from build123d import *

# Parameters (mm, degrees)
SKETCH2_W               = 8
SKETCH2_H               = 20
SKETCH2_W_2             = 11.75
SKETCH2_H_2             = 12.66
BOSS_EXTRUDE1_DEPTH     = 5
SKETCH3_W               = 13.1
SKETCH3_H               = 7
BOSS_EXTRUDE2_DEPTH     = 28
SKETCH4_W               = 5.75
SKETCH4_H               = 12.66
CUT_EXTRUDE1_DEPTH      = 62.587336361
SKETCH5_R               = 2
CUT_EXTRUDE2_DEPTH      = 61.902073035
SKETCH6_R               = 2
CUT_EXTRUDE3_DEPTH      = 60.059292241
SKETCH7_W               = 7
SKETCH7_H               = 28
BOSS_EXTRUDE3_DEPTH     = 19.4
SKETCH8_W               = 27
SKETCH8_H               = 33
BOSS_EXTRUDE4_DEPTH     = 2
SKETCH9_W               = 27
SKETCH9_H               = 33
BOSS_EXTRUDE5_DEPTH     = 2
CUT_EXTRUDE4_DEPTH      = 68.4388612
CUT_EXTRUDE4_DEPTH_BACK = 68.4388612


with BuildPart() as part:
    # Sketch2 → Boss-Extrude1 (new body)
    with BuildSketch(Plane(origin=(0, 0, 0), x_dir=(1, 0, 0), z_dir=(0, 1, 0))):
        with Locations((-4, 10)):
            Rectangle(SKETCH2_W, SKETCH2_H)
        Polygon((40, 0), (0, 0), (-8, 0), (-8, -7), (3.75, -7), (16.85, -7), (28.6, -7), (48, -7), (48, 0), align=None)
        with Locations((-2.125, -13.33)):
            Rectangle(SKETCH2_W_2, SKETCH2_H_2)
        with Locations((22.725, -13.33)):
            Rectangle(SKETCH2_W_2, SKETCH2_H_2)
        with Locations((44, 10)):
            Rectangle(SKETCH2_W, SKETCH2_H)
    extrude(amount=BOSS_EXTRUDE1_DEPTH)

    # Sketch3 → Boss-Extrude2 (add)
    with BuildSketch(Plane.XZ):
        Polygon((3.75, 19.66), (-8, 19.66), (-8, 0), (0, 0), (3.75, 0), (3.75, 7), align=None)
        with Locations((10.3, 3.5)):
            Rectangle(SKETCH3_W, SKETCH3_H)
        Polygon((16.85, 19.66), (16.85, 7), (16.85, 0), (28.6, 0), (28.6, 7), (28.6, 19.66), align=None)
    extrude(amount=BOSS_EXTRUDE2_DEPTH)

    # Sketch4 → Cut-Extrude1 (cut, through all)
    with BuildSketch(Plane.XZ.offset(28)):
        with Locations((-5.125, 13.33)):
            Rectangle(SKETCH4_W, SKETCH4_H)
        with Locations((25.725, 13.33)):
            Rectangle(SKETCH4_W, SKETCH4_H)
    extrude(amount=-CUT_EXTRUDE1_DEPTH, mode=Mode.SUBTRACT)

    # Sketch5 → Cut-Extrude2 (cut, through all)
    with BuildSketch(Plane.ZY.offset(2.25)):
        with Locations((13.33, -2)):
            Circle(SKETCH5_R)
        with Locations((13.33, -21)):
            Circle(SKETCH5_R)
        with Locations((13.33, -11.5)):
            Circle(SKETCH5_R)
    extrude(amount=-CUT_EXTRUDE2_DEPTH, mode=Mode.SUBTRACT)

    # Sketch6 → Cut-Extrude3 (cut, through all)
    with BuildSketch(Plane.XZ):
        with Locations(Location((43.95, -5, 0), (0, 0, 270))):
            Circle(SKETCH6_R)
        with Locations(Location((43.95, -15, 0), (0, 0, 270))):
            Circle(SKETCH6_R)
        with Locations(Location((-3.95, -5, 0), (0, 0, 270))):
            Circle(SKETCH6_R)
        with Locations(Location((-3.95, -15, 0), (0, 0, 270))):
            Circle(SKETCH6_R)
    extrude(amount=-CUT_EXTRUDE3_DEPTH, mode=Mode.SUBTRACT)

    # Sketch7 → Boss-Extrude3 (add)
    with BuildSketch(Plane(origin=(28.6, 0, 0), x_dir=(0, 0, -1), z_dir=(1, 0, 0))):
        with Locations((-3.5, -14)):
            Rectangle(SKETCH7_W, SKETCH7_H)
    extrude(amount=BOSS_EXTRUDE3_DEPTH)

    # Sketch8 → Boss-Extrude4 (add)
    with BuildSketch(Plane(origin=(48, 0, 0), x_dir=(0, 0, -1), z_dir=(1, 0, 0))):
        with Locations((6.5, -11.5)):
            Rectangle(SKETCH8_W, SKETCH8_H)
    extrude(amount=BOSS_EXTRUDE4_DEPTH)

    # Sketch9 → Boss-Extrude5 (add)
    with BuildSketch(Plane.ZY.offset(8)):
        with Locations((-6.5, -11.5)):
            Rectangle(SKETCH9_W, SKETCH9_H)
    extrude(amount=BOSS_EXTRUDE5_DEPTH)

    # Sketch10 → Cut-Extrude4 (cut, two sides: drawn at the far end of the back side and taken through both)
    with BuildSketch(Plane.ZY.offset(-48).offset(-CUT_EXTRUDE4_DEPTH_BACK)):
        Polygon((-20, 0), (0, -28), (-20, -28), align=None)
    extrude(amount=CUT_EXTRUDE4_DEPTH + CUT_EXTRUDE4_DEPTH_BACK, mode=Mode.SUBTRACT)


solid = part.part
The model under review builds one solid part; all positions refer to its coordinate system, in mm. A direction names the side the tool comes from. Give positions to 0.01 mm unless a question says otherwise; leave off trailing zeros. Order: outer loops, then holes, each group sorted by start corner. A loop starts at its lowest first (then second) coordinate and runs counter-clockwise, first axis right, second up. Notation, with made-up numbers: M 0,79.25 L 34,79.25 A22 cw 34,91.25 Z; hole C 0,20 d7. An arc over 180 degrees is marked long. Answer in a Markdown table with one row per item. Add a question column.
1. To check wall thickness, follow line 1 along X through (y, z) = (3.45, -5); line 2 along Y through (x, z) = (2.3, 13.33); line 3 along X through (y, z) = (-6.5, 15). State the ranges of each line that lie inside material, in increasing order.
2. Add section B-B on x = 43.95. State the section outline as (y, z) points, plus the area to 3 significant figures.
3. Add section C-C on y = -21. State the section outline as (x, z) points.
4. Add section A-A on z = -5. State the section outline as (x, y) points.
5. Mouldability with a two-part tool opening along Y and no side actions: class faces 4 (the cylindrical face through (0.708, -2.766, 15.177)), 5 (the flat face through (3.75, -11, 16)), 6 (the flat face through (49, -14, -10)) as released by +Y, released by -Y, zero draft, split by the parting line, or undercut.
6. Add section D-D on z = 17. State the section outline as (x, y) points, plus the area to 3 significant figures.
7. For pin 1 Ø4.5 at (y, z) = (-11.5, 13.33) entering from +X; pin 2 Ø5 at (x, y) = (19, -22) entering from -Z; pin 3 Ø3.5 at (y, z) = (-2, 13.33) entering from +X; pin 4 Ø4 at (x, z) = (-2, -5) entering from -Y, all flat-tipped, find the tip position at first contact; note any pin that passes through.
8. Machinability: for faces 1 (the flat face through (48, -11, -8)), 2 (the flat face through (22.85, -12, 16)), 3 (the flat face through (16.85, -11, 11)), which of the approach directions +Z, -Z, +X, -X, +Y, -Y give a long, thin tool a straight path to every point of the face, cutting with its end or side? Answer none if there is none.
The answers:
| question | item | result |
|---|---|---|
| 1 | line 1 | -10 to -5.95, -1.95 to 0, 40 to 41.95, 45.95 to 50 |
| 1 | line 2 | -28 to -23, -19 to -13.5, -9.5 to -4, 0 to 5 |
| 1 | line 3 | -2.25 to 3.75, 16.85 to 22.85 |
| 2 | outline | M -28,0 L 0,0 L 0,-3 L 5,-3 L 5,7 L -28,7 Z; M 0,-20 L 5,-20 L 5,-17 L 0,-17 Z; M 0,-13 L 5,-13 L 5,-7 L 0,-7 Z |
| 2 | area | 291 mm2 |
| 3 | outline | M -10,-5 L -8,-5 L -8,0 L 48,0 L 48,-5 L 50,-5 L 50,7 L 22.85,7 L 22.85,11.33 L 16.85,11.33 L 16.85,7 L 3.75,7 L 3.75,11.33 L -2.25,11.33 L -2.25,7 L -10,7 Z; M -2.25,15.33 L 3.75,15.33 L 3.75,19.66 L -2.25,19.66 Z; M 16.85,15.33 L 22.85,15.33 L 22.85,19.66 L 16.85,19.66 Z |
| 4 | outline | M -10,-21 L -8,-21 L -8,0 L -5.95,0 L -5.95,5 L -10,5 Z; M -1.95,0 L 0,0 L 0,5 L -1.95,5 Z; M 40,0 L 41.95,0 L 41.95,5 L 40,5 Z; M 45.95,0 L 48,0 L 48,-21 L 50,-21 L 50,5 L 45.95,5 Z |
| 5 | face 4 | undercut |
| 5 | face 5 | zero draft |
| 5 | face 6 | released by -Y |
| 6 | outline | M -2.25,-28 L 3.75,-28 L 3.75,5 L -2.25,5 Z; M 16.85,-28 L 22.85,-28 L 22.85,5 L 16.85,5 Z |
| 6 | area | 396 mm2 |
| 7 | pin 1 | x = 22.85 |
| 7 | pin 2 | z = 0 |
| 7 | pin 3 | through |
| 7 | pin 4 | y = 0 |
| 8 | face 1 | -Z, -Y |
| 8 | face 2 | +Z, +X, +Y, -Y |
| 8 | face 3 | +Z, +Y, -Y |
